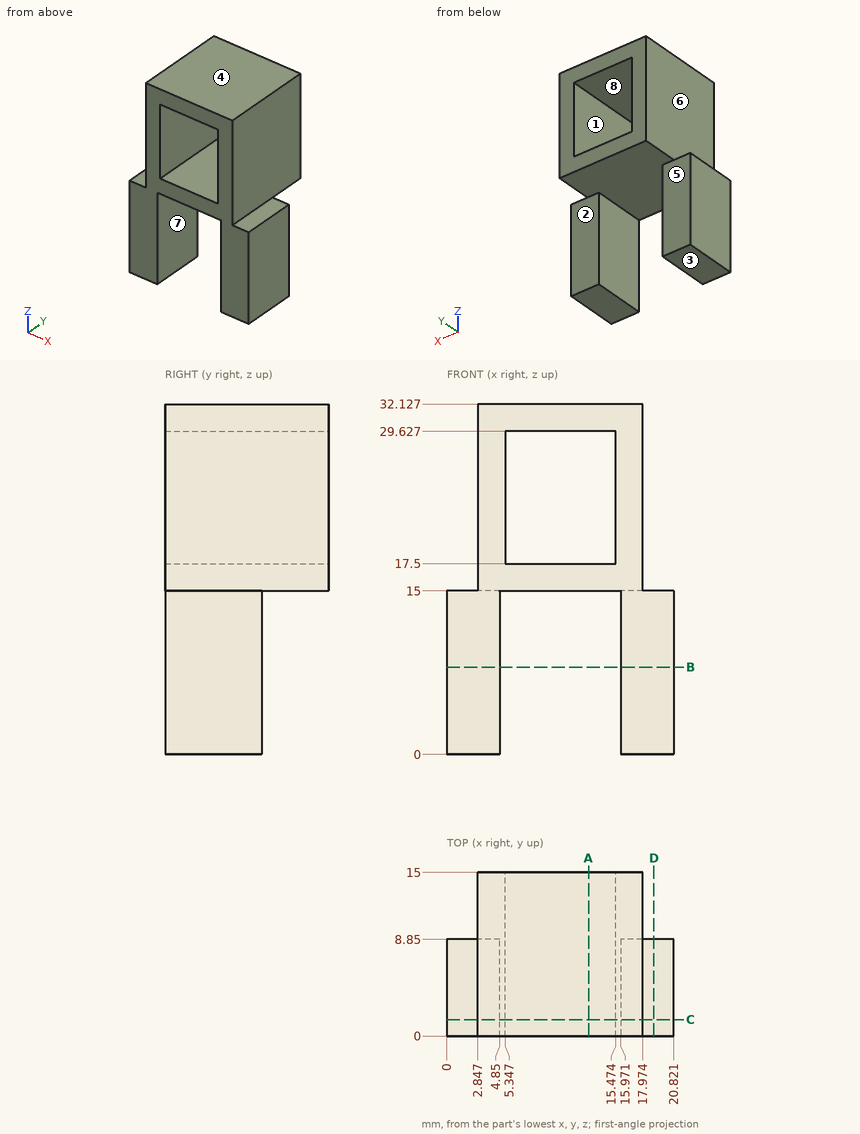
Geometry: see drawing. Coordinates: mm, zero at the bounding-box minimum. A direction names the side the tool comes from. Round coordinates to 2 decimals unless told otherwise and drop trailing zeros. Loops run counter-clockwise (first coordinate to the right, second up) from the corner with the lowest first, then second, coordinate; pieces in that order, holes last. Notation, with made-up numbers: M 46,59.25 L 86,59.25 A19 cw 86,90.25 Z; hole C 18,63.5 d4. An arc over 180 degrees is marked long. Use a Markdown table: item, result. Add a question column.
1. Set-up query: the marked faces 5, 6, 7 and 8. Return all of +Z, -Z, +X, -X, +Y, -Y with unobstructed straight access to the full face (end or side cutting, diameter ignored); none if empty.
2. Ray query, line 1 along X through (y, z) = (14.25, 27); line 2 along Z through (x, y) = (14.5, 7.25); line 3 along X through (y, z) = (3.25, 2). Return the intervals inside material, ascending. Write a range as [from, to].
3. Cut plane B-B, the plane z = 8. Output: boundary loops of the cut face in (x, y).
4. Contact query for flat-ended pins moving along their axis: pin 1 (6 mm diameter, centred on y = 4.5, z = 25.5, fed in from -X); pin 2 (5.5 mm diameter, centred on x = 3, z = 6.5, fed in from +Y); pin 3 (3.5 mm diameter, centred on y = 7.5, z = 21.5, fed in from +X); pin 4 (4 mm diameter, centred on x = 9, z = 12.5, fed in from -Y). Output: stop coordinate, or through.
5. Pull-direction query (Z, two-part tool) for the marked faces 1, 2, 3 and 4; classes: +Z half, -Z half, draft (parallel to the pull), parting line (faces both ways), or undercut.
6. Cut plane A-A, the plane x = 13. Output: boundary loops of the cut face in (y, z), and give its area (3 significant figures).
7. Cut plane D-D, the plane x = 19. Output: boundary loops of the cut face in (y, z), and give its area (3 significant figures).
8. Cut plane C-C, the plane y = 1.5. Output: boundary loops of the cut face in (x, z).
Solution:
| question | item | result |
|---|---|---|
| 1 | face 5 | -Z, +X, -X, +Y |
| 1 | face 6 | +Z, -X, +Y, -Y |
| 1 | face 7 | -Z, +Y, -Y |
| 1 | face 8 | +Y, -Y |
| 2 | line 1 | x = [2.85, 5.35], [15.47, 17.97] |
| 2 | line 2 | z = [15, 17.5], [29.63, 32.13] |
| 2 | line 3 | x = [0, 4.85], [15.97, 20.82] |
| 3 | outline | M 0,0 L 4.85,0 L 4.85,8.85 L 0,8.85 Z; M 15.97,0 L 20.82,0 L 20.82,8.85 L 15.97,8.85 Z |
| 4 | pin 1 | stops at x = 2.85 |
| 4 | pin 2 | stops at y = 8.85 |
| 4 | pin 3 | stops at x = 17.97 |
| 4 | pin 4 | passes through |
| 5 | face 1 | undercut |
| 5 | face 2 | draft |
| 5 | face 3 | -Z half |
| 5 | face 4 | +Z half |
| 6 | outline | M 0,15 L 15,15 L 15,17.5 L 0,17.5 Z; M 0,29.63 L 15,29.63 L 15,32.13 L 0,32.13 Z |
| 6 | area | 75.0 mm2 |
| 7 | outline | M 0,0 L 8.85,0 L 8.85,15 L 0,15 Z |
| 7 | area | 133 mm2 |
| 8 | outline | M 0,0 L 4.85,0 L 4.85,15 L 15.97,15 L 15.97,0 L 20.82,0 L 20.82,15 L 17.97,15 L 17.97,32.13 L 2.85,32.13 L 2.85,15 L 0,15 Z; hole M 5.35,17.5 L 15.47,17.5 L 15.47,29.63 L 5.35,29.63 Z |
